Verification items for the finished model (mm, model axes). A direction names the side the tool comes from. Round coordinates to 2 decimals unless told otherwise and drop trailing zeros. Loops run counter-clockwise (first coordinate to the right, second up) from the corner with the lowest first, then second, coordinate; pieces in that order, holes last. Notation, with made-up numbers: (-21, 42.5) -> (25, 42.5) arc R12 ccw to (25, 58.5) -> close; hole circle Ø1 at (56, 27). An arc over 180 degrees is marked (long way). Write item = value, one per line.
```python
from build123d import *

# Parameters (mm, degrees)
SKETCH024_R      = 6
EXTRUDE011_DEPTH = 150
EXTRUDE010_DEPTH = 30
SKETCH022_W      = 15
SKETCH022_H      = 79.05159
SKETCH022_H_2    = 80
EXTRUDE009_DEPTH = 150


with BuildPart() as extrude011:
    # Sketch024 → Extrude011 (new body, symmetric)
    with BuildSketch(Plane.YZ):
        Circle(SKETCH024_R)
    extrude(amount=EXTRUDE011_DEPTH, both=True)


with BuildPart() as extrude022:
    # Sketch023 → Extrude010 (new body, symmetric)
    with BuildSketch(Plane.XZ):
        with BuildLine():
            Line((30, 3), (30, -3))
            ThreePointArc((25, -8), (28.535534, -6.535534), (30, -3))
            Line((25, -8), (-25, -8))
            ThreePointArc((-30, -3), (-28.535534, -6.535534), (-25, -8))
            Line((-30, -3), (-30, 3))
            ThreePointArc((-25, 8), (-28.535534, 6.535534), (-30, 3))
            Line((-25, 8), (25, 8))
            ThreePointArc((30, 3), (28.535534, 6.535534), (25, 8))
        make_face()
    extrude(amount=EXTRUDE010_DEPTH, both=True)


with BuildPart() as extrude021:
    # Sketch022 → Extrude009 (new body, symmetric)
    with BuildSketch(Plane.YZ):
        with Locations((-18.5, 0.159191)):
            Rectangle(SKETCH022_W, SKETCH022_H)
        with Locations((18.5, -0.315014)):
            Rectangle(SKETCH022_W, SKETCH022_H_2)
    extrude(amount=EXTRUDE009_DEPTH, both=True)


with BuildPart() as obj1:
    # Sketch021 → Revolve001 (revolve)
    with BuildSketch(Plane.XZ):
        Polygon((-50, 0), (-50, 11), (-30, 15), (30, 15), (50, 11), (50, 0), align=None)
    revolve(axis=Axis((-50, 0, 0), (-1, 0, 0)))

    # Cut009: cut Extrude021
    add(extrude021.part, mode=Mode.SUBTRACT)

    # Cut010: cut Extrude022
    add(extrude022.part, mode=Mode.SUBTRACT)

    # Cut011: cut Extrude011
    add(extrude011.part, mode=Mode.SUBTRACT)


with BuildPart() as obj1_1:
    # Cut011 placement: moved
    add(obj1.part.moved(Location((-180, 0, 0))))


solid = obj1_1.part
```
(1) Sectioned sample at C-C, the plane x = -215. Record the cut outline in (y, z), and give its area (3 significant figures).
Filled sheet:
outline = (-11, -8.66) arc R14 ccw to (11, -8.66) -> (11, 8.66) arc R14 ccw to (-11, 8.66) -> close; hole circle Ø12 at (0, 0)
area = 432 mm2
(2) Set-up check for faces 1 (the face through (-150, 8, 0)), 2 (the face through (-140, -6, 0)): record each of +Z, -Z, +X, -X, +Y, -Y from which the full face is reachable in a straight line by a thin tool's end or side.
Filled sheet:
face_1 = +Y, -Y
face_2 = +X, -X
(3) Sectioned sample at B-B, the plane y = 0. Record the cut outline in (x, z), and give its area (3 significant figures).
Filled sheet:
outline = (-230, -11) -> (-210, -15) -> (-150, -15) -> (-130, -11) -> (-130, -6) -> (-151, -6) arc R5 cw to (-155, -8) -> (-205, -8) arc R5 cw to (-209, -6) -> (-230, -6) -> close; (-230, 6) -> (-209, 6) arc R5 cw to (-205, 8) -> (-155, 8) arc R5 cw to (-151, 6) -> (-130, 6) -> (-130, 11) -> (-150, 15) -> (-210, 15) -> (-230, 11) -> close
area = 1,420 mm2
(4) Sectioned sample at A-A, the plane x = -167. Record the cut outline in (y, z).
Filled sheet:
outline = (-11, -10.2) arc R15 ccw to (11, -10.2) -> (11, -8) -> (-11, -8) -> close; (-11, 8) -> (11, 8) -> (11, 10.2) arc R15 ccw to (-11, 10.2) -> close
(5) Draft check along Y on faces 3 (the face through (-208, 0, 7)), 4 (the face through (-219, -6, 0)), 5 (the face through (-222.08, 0.28, -12.58)). Enter one of: released by +Y, released by -Y, zero draft, split by the parting line, or undercut.
Filled sheet:
face_3 = zero draft
face_4 = undercut
face_5 = split by the parting line
(6) Material ranges on probe 1 along Y at (x, z) = (-141.25, 0); probe 2 along Z at (x, y) = (-169.5, 3.25); probe 3 along Z at (x, y) = (-220, 0), recorded low to high. Write a range as from..to.
Filled sheet:
probe_1 = -11..-6, 6..11
probe_2 = -14.64..-8, 8..14.64
probe_3 = -13..-6, 6..13
(7) Go/stop test with flat-tipped pins: pin 1 Ø2 at (x, y) = (-216, 6) entering from +Z; pin 2 Ø1 at (x, y) = (-182, -8.5) entering from +Z; pin 3 Ø8 at (x, y) = (-166.5, 5.5) entering from +Z. Record where each tip stops, or that it passes through.
Filled sheet:
pin_1 = 12.92
pin_2 = 12.69
pin_3 = 14.92
